Model file for the job. Use its own axes, mm. A direction names the side the tool comes from. Round coordinates to 2 decimals unless told otherwise and drop trailing zeros. Loops run counter-clockwise (first coordinate to the right, second up) from the corner with the lowest first, then second, coordinate; pieces in that order, holes last. Notation, with made-up numbers: M 30,-35 L 81,-35 A21 cw 81,-10 Z; hole C 8,8.25 d2. An arc over 180 degrees is marked long. Use a Markdown table: item, result. Add a question column.
Q1. Cut at C-C (z = 27). Give the cut face in (x, y) (3 decimals), plus the area to 3 significant figures.
Q2. Pin check, flat tips, straight feed: pin 1 (2.5 mm diameter, centred on x = -30.5, y = -23.5, fed in from -Z); pin 2 (5 mm diameter, centred on y = -0.5, z = 34, fed in from -X) (3 decimals); pin 3 (5 mm diameter, centred on y = 3.5, z = 17.5, fed in from -X) (3 decimals); pin 4 (14.5 mm diameter, centred on x = -6, z = 23, fed in from -Y) (3 decimals). Stop position of each tip, or through.
Q3. Tool access for faces 5 (the face through (30.06, -4.63, 21.34)), 6 (the face through (-17.49, -17.57, 4.37)), 7 (the face through (22, 23, 2.7)), 8 (the face through (-30.062, -4.194, 21.774)), 9 (the face through (17.03, -23.04, 4.37)): list every direction of +Z, -Z, +X, -X, +Y, -Y with a clear straight run to the whole face (end or side of a thin tool).
Q4. Cut at D-D (y = 0). Give the cut face in (x, z) (3 decimals).
Q5. Mould opens along Z. For faces 1 (the face through (-27.53, 6.62, 35.45)), 2 (the face through (25.625, 11, 22)), 3 (the face through (-23, 23, 2.7)), 4 (the face through (-30.06, 9.71, 38.55)) say: +Z half, -Z half, draft (parallel to the pull), parting line (faces both ways), or undercut.
Q6. Cut at B-B (x = 21.5). Give the cut face in (y, z) (3 decimals), plus the area to 3 significant figures.
Q7. Probe line 1 (X direction, y = -12, z = 8.5) (3 decimals); line 2 (X direction, y = -20.5, z = 0.6) (3 decimals). List the from-to ranges inside material, lowest first. Write a range as from..to.
Q8. Cut at A-A (y = 12). Give the cut face in (x, z) (3 decimals).
from build123d import *

# Parameters (mm, degrees)
F0_W      = 51.25
F0_H      = 51.25
F0_R      = 2.3
F0_R_2    = 24
F1_DEPTH  = 6
F3_DEPTH  = 3.3
F4_W      = 51.25
F4_H      = 51.25
F4_W_2    = 48.25
F4_H_2    = 48.25
F5_DEPTH  = 55
F7_DEPTH  = 51.251
F9_DEPTH  = 9
F11_DEPTH = 9
F12_R     = 1.75
F13_DEPTH = 40.482863


with BuildPart() as f1:
    # F0 (on Top) → F1 (new body)
    with BuildSketch(Plane.XY):
        Rectangle(F0_W, F0_H)
        with Locations((-20.5, -20.5)):
            Circle(F0_R, mode=Mode.SUBTRACT)
        with Locations((20.5, -20.5)):
            Circle(F0_R, mode=Mode.SUBTRACT)
        with Locations((-20.5, 20.5)):
            Circle(F0_R, mode=Mode.SUBTRACT)
        Circle(F0_R_2, mode=Mode.SUBTRACT)
        with Locations((20.5, 20.5)):
            Circle(F0_R, mode=Mode.SUBTRACT)
    extrude(amount=F1_DEPTH)

    # F2 (on face) → F3 (cut)
    with BuildSketch(Plane.XY.offset(6)):
        Polygon((-25.625, 25.625), (-25.625, 19.614592), (-20.535355, 14.524948), (-14.524948, 20.535355), (-19.614592, 25.625), align=None)
        Polygon((19.614592, 25.625), (14.524948, 20.535355), (20.535355, 14.524948), (25.625, 19.614592), (25.625, 25.625), align=None)
        Polygon((25.625, -25.625), (25.625, -19.614592), (20.535355, -14.524948), (14.524948, -20.535355), (19.614592, -25.625), align=None)
        Polygon((-14.524948, -20.535355), (-20.535355, -14.524948), (-25.625, -19.614592), (-25.625, -25.625), (-19.614592, -25.625), align=None)
    extrude(amount=-F3_DEPTH, mode=Mode.SUBTRACT)

    # F4 (on face) → F5 (join)
    with BuildSketch(Plane.XY.offset(6)):
        Rectangle(F4_W, F4_H)
        Rectangle(F4_W_2, F4_H_2, mode=Mode.SUBTRACT)
    extrude(amount=F5_DEPTH)

    # F6 (on face) → F7 (cut, through all)
    with BuildSketch(Plane.YZ.offset(25.625)):
        Polygon((-25.625, 61), (-25.625, 6), (25.625, 57.25), (25.625, 61), align=None)
    extrude(amount=-F7_DEPTH, mode=Mode.SUBTRACT)

    # F8 (on face) → F9 (join)
    with BuildSketch(Plane.YZ.offset(25.625)):
        Polygon((8.316125, 39.941125), (-25.625, 6), (-19.968146, 6), (11.144553, 37.112698), align=None)
    extrude(amount=F9_DEPTH)

    # F10 (on face) → F11 (join)
    with BuildSketch(Plane(origin=(-25.625, 0, 0), x_dir=(0, -1, 0), z_dir=(-1, 0, 0))):
        Polygon((19.968146, 6), (25.625, 6), (-8.316125, 39.941125), (-11.144553, 37.112698), align=None)
    extrude(amount=F11_DEPTH)

    # F12 (on face) → F13 (cut, through all)
    with BuildSketch(Plane(origin=(0, -15.8125, 15.8125), x_dir=(1, 0, 0), z_dir=(0, -0.707107, 0.707107))):
        with Locations((29.2, 29.223029)):
            Circle(F12_R)
        with Locations((29.2, -8.976971)):
            Circle(F12_R)
        with Locations((-29.2, 29.223029)):
            Circle(F12_R)
        with Locations((-29.2, -8.976971)):
            Circle(F12_R)
    extrude(amount=-F13_DEPTH, mode=Mode.SUBTRACT)


solid = f1.part
Checked values:
| question | item | result |
|---|---|---|
| 1 | outline | M -34.625,-4.625 L -24.125,-4.625 L -24.125,24.125 L 24.125,24.125 L 24.125,-4.625 L 34.625,-4.625 L 34.625,1.032 L 25.625,1.032 L 25.625,25.625 L -25.625,25.625 L -25.625,1.032 L -34.625,1.032 Z |
| 1 | area | 265 mm^2 |
| 2 | pin 1 | stops at z = 6 |
| 2 | pin 2 | stops at x = -34.625 |
| 2 | pin 3 | stops at x = -25.625 |
| 2 | pin 4 | stops at y = 24.125 |
| 3 | face 5 | -Z, +X, +Y |
| 3 | face 6 | +Z |
| 3 | face 7 | none |
| 3 | face 8 | -Z, -X, +Y |
| 3 | face 9 | +X |
| 4 | outline | M -34.625,25.968 L -25.625,25.968 L -25.625,0 L -24,0 L -24,6 L -24.125,6 L -24.125,31.625 L -34.625,31.625 Z; M 24,0 L 25.625,0 L 25.625,25.968 L 34.625,25.968 L 34.625,31.625 L 24.125,31.625 L 24.125,6 L 24,6 Z |
| 5 | face 1 | undercut |
| 5 | face 2 | draft |
| 5 | face 3 | undercut |
| 5 | face 4 | +Z half |
| 6 | outline | M -25.625,0 L -22.571,0 L -22.571,2.7 L -25.625,2.7 Z; M -25.625,6 L -24.125,6 L -24.125,7.5 Z; M -18.429,0 L -10.665,0 L -10.665,6 L -15.49,6 L -15.49,2.7 L -18.429,2.7 Z; M 10.665,0 L 18.429,0 L 18.429,2.7 L 15.49,2.7 L 15.49,6 L 10.665,6 Z; M 22.571,0 L 25.625,0 L 25.625,2.7 L 22.571,2.7 Z; M 24.125,6 L 25.625,6 L 25.625,57.25 L 24.125,55.75 Z |
| 6 | area | 167 mm^2 |
| 7 | line 1 | x = -25.625..-24.125, 24.125..25.625 |
| 7 | line 2 | x = -25.625..-22.8, -18.2..-12.48, 12.48..18.2, 22.8..25.625 |
| 8 | outline | M -25.625,0 L -20.785,0 L -20.785,6 L -24.125,6 L -24.125,43.625 L -25.625,43.625 Z; M 20.785,0 L 25.625,0 L 25.625,43.625 L 24.125,43.625 L 24.125,6 L 20.785,6 Z |
